Design review of the part built by this model. Coordinates are the model's own, in mm. Face numbers are marked on the shaded views. A direction names the side the tool comes from. Give positions to 0.01 mm unless a question says otherwise; leave off trailing zeros. Write each loop counter-clockwise with the first axis right and the second up, starting at its lowest first coordinate (ties: lowest second). Pieces come first, ordered by that corner, then holes. Notation, with made-up numbers: (79.5, 70) -> (95.5, 70) arc R20 cw to (95.5, 91) -> close; hole circle Ø2 at (31, 5). An arc over 180 degrees is marked (long way). Use CSV: the item, a comma, the result in double quotes.
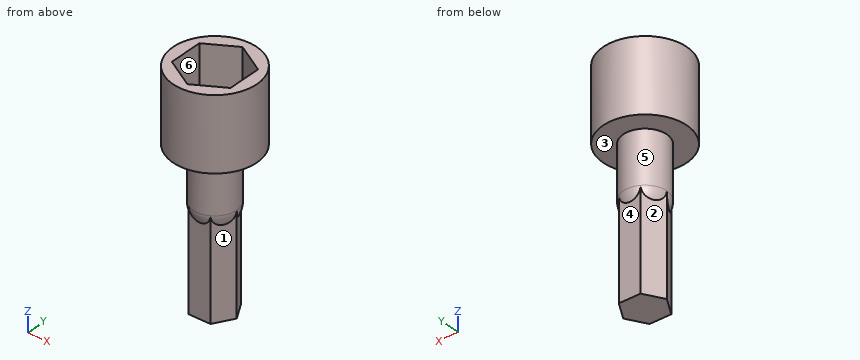
```python
from build123d import *

# Parameters (mm, degrees)
F0_R     = 6.9596
F1_DEPTH = 12.0904
F3_DEPTH = 8.636
F5_DEPTH = 25.4


with BuildPart() as f1:
    # F0 (on Top) → F1 (new body)
    with BuildSketch(Plane.XY):
        Circle(F0_R)
    extrude(amount=F1_DEPTH)

    # F2 (on face) → F3 (cut)
    with BuildSketch(Plane.XY.offset(12.0904)):
        Polygon((4.8768, -2.815622), (4.8768, 2.815622), (0, 5.631244), (-4.8768, 2.815622), (-4.8768, -2.815622), (0, -5.631244), align=None)
    extrude(amount=-F3_DEPTH, mode=Mode.SUBTRACT)

    # F4 (on face) → F5 (join)
    with BuildSketch(Plane(origin=(0, 0, 0), x_dir=(1, 0, 0), z_dir=(0, 0, -1))):
        Polygon((-1.81109, -3.1369), (1.81109, -3.1369), (3.62218, 0), (1.81109, 3.1369), (-1.81109, 3.1369), (-3.62218, 0), align=None)
    extrude(amount=F5_DEPTH)

    # F6 (on Front) → F7 (revolve)
    with BuildSketch(Plane.XZ):
        with BuildLine():
            Line((0, 0), (-3.62218, 0))
            Line((-3.62218, 0), (-3.62218, -8.7122))
            ThreePointArc((-3.62218, -8.7122), (-2.561268, -11.273468), (0, -12.33438))
            Line((0, -12.33438), (0, 0))
        make_face()
    revolve(axis=Axis((0, 0, -6.16719), (0, 0, -1)))


solid = f1.part
```
(1) Take a section at A-A (y = 4.25). Write out the cut boundary in (x, z).
Established:
outline,"(-5.51, 0) -> (5.51, 0) -> (5.51, 12.09) -> (2.39, 12.09) -> (2.39, 3.45) -> (-2.39, 3.45) -> (-2.39, 12.09) -> (-5.51, 12.09) -> close"
(2) Mouldability with a two-part tool opening along Y and no side actions: class the marked faces 4, 5 and 6 as +Y half, -Y half, draft (parallel to the pull), parting line (faces both ways), or undercut.
Established:
face 4,"+Y half"
face 5,"parting line"
face 6,"undercut"
(3) For line 1 along Y through (x, z) = (0.25, -12); line 2 along Z through (x, y) = (2.25, -2.25); line 3 along X through (y, z) = (-1.75, 8), list the stretches that pass through material, from the lowest coordinate up. Write a range as [from, to].
Established:
line 1,"y = [-3.14, 3.14]"
line 2,"z = [-25.4, 3.45]"
line 3,"x = [-6.74, -4.88], [4.88, 6.74]"
(4) Take a section at D-D (y = -5). Write out the cut boundary in (x, z), then the cut area to 3 significant figures.
Established:
outline,"(-4.84, 0) -> (4.84, 0) -> (4.84, 12.09) -> (1.09, 12.09) -> (1.09, 3.45) -> (-1.09, 3.45) -> (-1.09, 12.09) -> (-4.84, 12.09) -> close"
area,"98.2 mm2"
(5) Take a section at B-B (z = -16). Write out the cut boundary in (x, y), then the cut area to 3 significant figures.
Established:
outline,"(-3.62, 0) -> (-1.81, -3.14) -> (1.81, -3.14) -> (3.62, 0) -> (1.81, 3.14) -> (-1.81, 3.14) -> close"
area,"34.1 mm2"
(6) Tool access review of the marked faces 1, 2 and 3: name each direction out of +Z, -Z, +X, -X, +Y, -Y from which nothing blocks a thin tool from reaching the whole face with its end or side.
Established:
face 1,"-Z, +X, -Y"
face 2,"-Z, -X, +Y"
face 3,"-Z"
(7) Clearance check with flat-ended pins moving along their axes: pin 1 (3 mm diameter, centred on y = -0.5, z = 6.5, fed in from -X); pin 2 (4 mm diameter, centred on x = -5, z = 8, fed in from -Y); pin 3 (1 mm diameter, centred on x = -5, y = -1.5, fed in from -Z); pin 4 (1.8 mm diameter, centred on x = -0.5, z = -16, fed in from +Y). State where each tip first meets the part, or that it passes through.
Established:
pin 1,"stops at x = -6.96"
pin 2,"stops at y = -6.28"
pin 3,"stops at z = 0"
pin 4,"stops at y = 3.14"
(8) Take a section at C-C (z = -3). Write out the cut boundary in (x, y).
Established:
outline,"circle Ø7.24 at (0, 0)"
